Can you work these out from the model? Positions are in its coordinate system, mm. Coordinates: 2 decimals unless noted, no trailing zeros. Order: outer loops, then holes, each group sorted by start corner. A loop starts at its lowest first (then second) coordinate and runs counter-clockwise, first axis right, second up. Notation, with made-up numbers: M -1.5,23 L 35.5,23 A11 cw 35.5,33 Z; hole C 79,83.25 d8. An arc over 180 degrees is marked long. Answer as CSV lines item,"result". Start each with the question number.
1. If we section it at D-D (x = -14): List the corners of the cut face in (y, z) for me, plus the area to 3 significant figures.
2. If we section it at B-B (z = 24.13): List the corners of the cut face in (x, y) for me (3 decimals), plus the area to 3 significant figures.
3. If we section it at A-A (x = 0): List the corners of the cut face in (y, z) for me (3 decimals), plus the area to 3 significant figures.
4. If we section it at C-C (z = -31): List the corners of the cut face in (x, y) for me (3 decimals), plus the area to 3 significant figures.
5. I need wall thicknesses on line 1 along X through (y, z) = (-5.25, 7.5); line 2 along X through (y, z) = (-2.5, -5.5); line 3 along Z through (x, y) = (0, -4.5) (3 decimals). Which ranges of each line are inside material? Lowest first, please. Write a range as from..to.
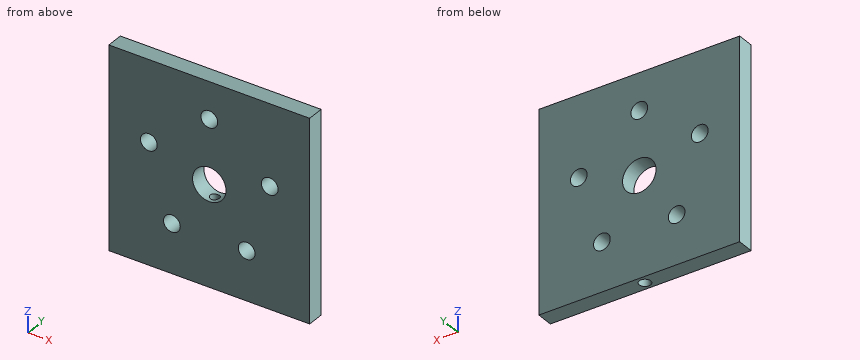
```python
from build123d import *

# Parameters (mm, degrees)
F0_W     = 76.2
F0_H     = 76.2
F0_R     = 3.175
F0_R_2   = 6.35
F1_DEPTH = 6.35
F2_R     = 2.15265
F3_DEPTH = 25.4
F4_R     = 1.7272
F5_REACH = 81.0862593299


with BuildPart() as f1:
    # F0 (on Front) → F1 (new body)
    with BuildSketch(Plane.XZ):
        Rectangle(F0_W, F0_H)
        with Locations((-14.1832581378, -19.5215800743)):
            Circle(F0_R, mode=Mode.SUBTRACT)
        with Locations((14.1832581378, -19.5215800743)):
            Circle(F0_R, mode=Mode.SUBTRACT)
        with Locations((-22.9489937382, 7.4565800743)):
            Circle(F0_R, mode=Mode.SUBTRACT)
        Circle(F0_R_2, mode=Mode.SUBTRACT)
        with Locations((22.9489937382, 7.4565800743)):
            Circle(F0_R, mode=Mode.SUBTRACT)
        with Locations((0, 24.13)):
            Circle(F0_R, mode=Mode.SUBTRACT)
    extrude(amount=F1_DEPTH)

    # F2 (on face) → F3 (cut)
    with BuildSketch(Plane(origin=(0, 0, -38.1), x_dir=(1, 0, 0), z_dir=(0, 0, -1))):
        with Locations((0, 3.175)):
            Circle(F2_R)
    extrude(amount=-F3_DEPTH, mode=Mode.SUBTRACT)

    f5_end = f1.faces().sort_by_distance((-6.35, -3.175, 0))[0]
    # F4 (on face) → F5 (cut, up to a face of the model that its end follows)
    with BuildSketch(Plane(origin=(0, 0, -38.1), x_dir=(1, 0, 0), z_dir=(0, 0, -1))):
        with Locations((0, 3.175)):
            Circle(F4_R)
    f5_long = extrude(amount=-F5_REACH, mode=Mode.PRIVATE)
    add(split(f5_long, bisect_by=f5_end, keep=Keep.ALL, mode=Mode.PRIVATE).solids().sort_by_distance((0, -3.175, -38.1))[0], mode=Mode.SUBTRACT)


solid = f1.part
```
Solved:
1,outline,"M -6.35,-38.1 L 0,-38.1 L 0,-22.69 L -6.35,-22.69 Z; M -6.35,-16.35 L 0,-16.35 L 0,38.1 L -6.35,38.1 Z"
1,area,"444 mm²"
2,outline,"M -38.1,-6.35 L -3.175,-6.35 L -3.175,0 L -38.1,0 Z; M 3.175,-6.35 L 38.1,-6.35 L 38.1,0 L 3.175,0 Z"
2,area,"444 mm²"
3,outline,"M -6.35,-38.1 L -5.328,-38.1 L -5.328,-12.7 L -4.902,-12.7 L -4.902,-6.35 L -6.35,-6.35 Z; M -6.35,6.35 L 0,6.35 L 0,20.955 L -6.35,20.955 Z; M -6.35,27.305 L 0,27.305 L 0,38.1 L -6.35,38.1 Z; M -1.448,-12.7 L -1.022,-12.7 L -1.022,-38.1 L 0,-38.1 L 0,-6.35 L -1.448,-6.35 Z"
3,area,"232 mm²"
4,outline,"M -38.1,-6.35 L 38.1,-6.35 L 38.1,0 L -38.1,0 Z; hole C 0,-3.175 d4.305"
4,area,"469 mm²"
5,line 1,"-38.1..-26.12, -19.77..19.77, 26.12..38.1"
5,line 2,"-38.1..-3.17, 3.17..38.1"
5,line 3,"6.35..20.955, 27.305..38.1"
